Could you check a few things on this model? Use its own coordinates, in mm. Face numbers are marked on the shaded views. A direction names the side the tool comes from. Coordinates: 2 decimals unless noted, no trailing zeros. Loops run counter-clockwise (first coordinate to the right, second up) from the corner with the lowest first, then second, coordinate; pieces in that order, holes last. Notation, with made-up numbers: (49.25, 76) -> (73.25, 76) arc R22 cw to (73.25, 101) -> close; hole circle Ø1 at (-16, 4). An arc over 180 degrees is marked (long way). One line per question, with ' | ' between items.
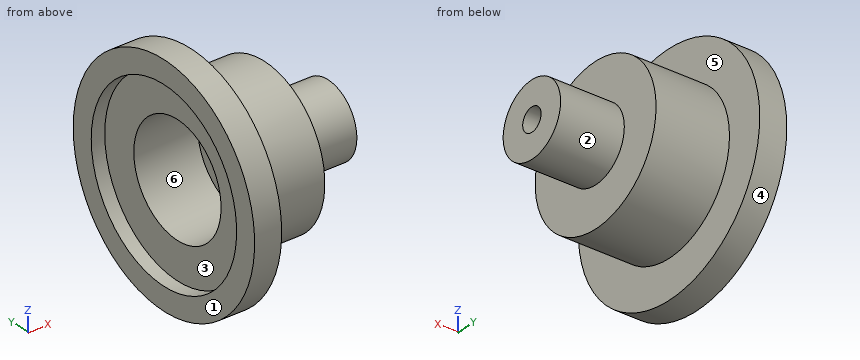
Autodesk Inventor part; units mm, degrees
ref_plane "YZ Plane" through (0, 0, 0) normal (1, 0, 0) x (0, 1, 0)
ref_plane "XZ Plane" through (0, 0, 0) normal (0, 1, 0) x (-1, 0, 0)
ref_plane "XY Plane" through (0, 0, 0) normal (0, 0, 1) x (1, 0, 0)
sketch "Sketch1" plane through (0, 0, 0) normal (0, 0, 1) x (1, 0, 0)
  line L0 (0, 4.75) -> (0, 5.925)
  line L1 (0, 5.925) -> (1.4, 5.925)
  line L2 (1.4, 5.925) -> (1.4, 3.95)
  line L3 (1.4, 3.95) -> (5.2, 3.95)
  line L4 (5.2, 3.95) -> (5.2, 1.875)
  line L5 (5.2, 1.875) -> (8.5, 1.875)
  line L6 (8.5, 1.875) -> (8.5, 0)
  line L7 (8.5, 0) -> (0, 0)
  line L8 (0, 4.75) -> (0.7, 4.75)
  line L9 (0.7, 4.75) -> (0.7, 2.85)
  line L10 (0.7, 2.85) -> (4, 2.85)
  line L11 (4, 2.85) -> (4, 0)
  dimension "d0" = 8.5
  dimension "d1" = 11.85
  dimension "d2" = 1.4
  dimension "d3" = 5.2
  dimension "d4" = 7.9
  dimension "d5" = 3.75
  dimension "d6" = 9.5
  dimension "d7" = 5.7
  dimension "d8" = 0.7
  dimension "d9" = 4
revolve "Revolution1" add sketch "Sketch1" angle 360 about axis through (8.5, 0, 0) along (-1, 0, 0)
hole "Hole1" at (8.5, 0, 0) direction (-1, 0, 0) diameter 1.2 end through all
properties part number "Hitec HS-225MG gear 3"
1) I need wall thicknesses on line 1 along Y through (x, z) = (5.85, 0) (3 decimals); line 2 along Z through (x, y) = (3.1, 0). Which ranges of each line are inside material? Lowest first, please. Write a range as from..to.
Data:
line 1: -1.875..-0.6, 0.6..1.875 | line 2: -3.95..-2.85, 2.85..3.95
2) I'm going to push flat-ended pins straight in: pin 1 Ø5 at (y, z) = (-0.5, -1) entering from -X; pin 2 Ø3 at (y, z) = (0.5, -1) entering from -X; pin 3 Ø6 at (y, z) = (-3, -4) entering from +X. Where does each tip first touch, or does it pass through?
Data:
pin 1: x = 0.7 | pin 2: x = 4 | pin 3: x = 5.2
3) If we section it at C-C on x = 5: Please give me the cut outline in (y, z), and give its area (3 significant figures).
Data:
outline: circle Ø7.9 at (0, 0); hole circle Ø1.2 at (0, 0) | area: 47.9 mm²
4) We'd pull the mould along Z, two halves only. Please class the marked faces 1, 2 and 3: pulls with the +Z half, pulls with the -Z half, needs draft (parallel to the pull), parting line crosses it, or undercut.
Data:
face 1: needs draft | face 2: parting line crosses it | face 3: undercut
5) If we section it at A-A on y = 0: Please give me the cut outline in (x, z) (3 decimals).
Data:
outline: (0, -5.925) -> (1.4, -5.925) -> (1.4, -3.95) -> (5.2, -3.95) -> (5.2, -1.875) -> (8.5, -1.875) -> (8.5, -0.6) -> (4, -0.6) -> (4, -2.85) -> (0.7, -2.85) -> (0.7, -4.75) -> (0, -4.75) -> close; (0, 4.75) -> (0.7, 4.75) -> (0.7, 2.85) -> (4, 2.85) -> (4, 0.6) -> (8.5, 0.6) -> (8.5, 1.875) -> (5.2, 1.875) -> (5.2, 3.95) -> (1.4, 3.95) -> (1.4, 5.925) -> (0, 5.925) -> close
6) If we section it at D-D on z = 1.25: Please give me the cut outline in (x, y), and give its area (3 significant figures).
Data:
outline: (0, -5.79) -> (1.4, -5.79) -> (1.4, -3.75) -> (5.2, -3.75) -> (5.2, -1.4) -> (8.5, -1.4) -> (8.5, 1.4) -> (5.2, 1.4) -> (5.2, 3.75) -> (1.4, 3.75) -> (1.4, 5.79) -> (0, 5.79) -> (0, 4.58) -> (0.7, 4.58) -> (0.7, 2.56) -> (4, 2.56) -> (4, -2.56) -> (0.7, -2.56) -> (0.7, -4.58) -> (0, -4.58) -> close | area: 30.6 mm²
7) On a 3-axis mill with a long thin cutter (end or side, diameter ignored), from which of +Z, -Z, +X, -X, +Y, -Y can I reach the whole of each face in a straight line? I mean the marked faces 4, 5 and 6. Say none if no direction works.
Data:
face 4: +X, -X | face 5: +X | face 6: -X
